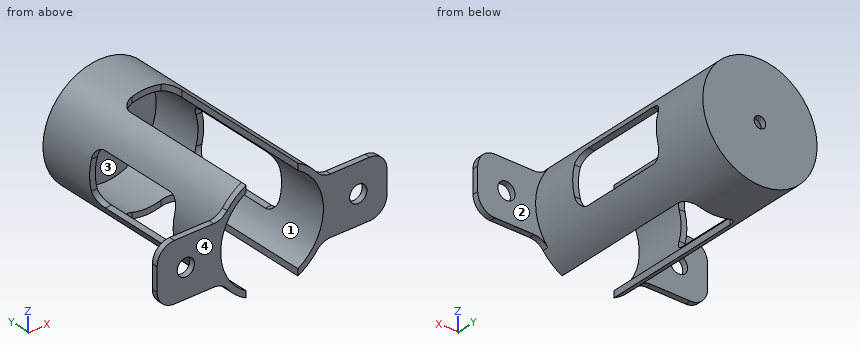
from build123d import *

# Parameters (mm, degrees)
SKETCH2_R           = 9.9375
BOSS_EXTRUDE1_DEPTH = 35.384
SKETCH4_R           = 1
CUT_EXTRUDE2_DEPTH  = 39.072762817
BOSS_EXTRUDE2_START = 1
SKETCH11_R          = 8.9375
BOSS_EXTRUDE2_DEPTH = 1
SKETCH12_R          = 8.9375
CUT_EXTRUDE7_DEPTH  = 34.384
CUT_EXTRUDE8_START  = -1
CUT_EXTRUDE8_DEPTH  = 26.538
SKETCH14_W          = 9
SKETCH14_H          = 17.692
CUT_EXTRUDE9_DEPTH  = 63.054664307
FILLET3_R           = 2
FILLET4_R           = 3
CUT_EXTRUDE10_REACH = 43.842
SKETCH15_R          = 1.5


# Read off the part's stored shape, not the designer's step: Cut-Extrude8
with BuildPart() as part:
    # Sketch2 → Boss-Extrude1 (new body)
    with BuildSketch(Plane(origin=(0, 0, 0), x_dir=(1, 0, 0), z_dir=(0, 1, 0))):
        with Locations(Location((0, 0, 0), (0, 0, 270))):
            Circle(SKETCH2_R)
    extrude(amount=BOSS_EXTRUDE1_DEPTH)

    # Sketch4 → Cut-Extrude2 (cut, through all)
    with BuildSketch(Plane(origin=(0, 35.384, 0), x_dir=(1, 0, 0), z_dir=(0, 1, 0))):
        with Locations(Location((0, 0, 0), (0, 0, 270))):
            Circle(SKETCH4_R)
    extrude(amount=-CUT_EXTRUDE2_DEPTH, mode=Mode.SUBTRACT)

    # Sketch11 → Boss-Extrude2 (add)
    with BuildSketch(Plane.XZ.offset(BOSS_EXTRUDE2_START)):
        with BuildLine():
            Line((8.588009446, 5), (20, 5))
            Line((20, 5), (20, -5))
            Line((20, -5), (8.588009446, -5))
            ThreePointArc((8.588009446, -5), (0, -9.9375), (-8.588009446, -5))
            Line((-8.588009446, -5), (-20, -5))
            Line((-20, -5), (-20, 5))
            Line((-20, 5), (-8.588009446, 5))
            ThreePointArc((-8.588009446, 5), (0, 9.9375), (8.588009446, 5))
        make_face()
        with Locations(Location((0, 0, 0), (0, 0, 270))):
            Circle(SKETCH11_R, mode=Mode.SUBTRACT)
    extrude(amount=-BOSS_EXTRUDE2_DEPTH)

    # Sketch12 → Cut-Extrude7 (cut)
    with BuildSketch(Plane.XZ):
        with Locations(Location((0, 0, 0), (0, 0, 270))):
            Circle(SKETCH12_R)
    extrude(amount=-CUT_EXTRUDE7_DEPTH, mode=Mode.SUBTRACT)

    # Cut-Extrude8 outline → Cut-Extrude8 (cut)
    with BuildSketch(Plane(origin=(0, 0, 0), x_dir=(1, 0, 0), z_dir=(0, 1, 0)).offset(CUT_EXTRUDE8_START)):
        with BuildLine():
            ThreePointArc((4.5, -7.721975541), (0, -8.9375), (-4.5, -7.721975541))
            Line((-4.5, -7.721975541), (-4.5, -8.860243013))
            ThreePointArc((-4.5, -8.860243013), (0, -9.9375), (4.5, -8.860243013))
            Line((4.5, -8.860243013), (4.5, -7.721975541))
        make_face()
        with BuildLine():
            Line((-4.5, 8.860243013), (-4.5, 7.721975541))
            ThreePointArc((-4.5, 7.721975541), (0, 8.9375), (4.5, 7.721975541))
            Line((4.5, 7.721975541), (4.5, 8.860243013))
            ThreePointArc((4.5, 8.860243013), (0, 9.9375), (-4.5, 8.860243013))
        make_face()
    extrude(amount=CUT_EXTRUDE8_DEPTH, mode=Mode.SUBTRACT)

    # Sketch14 → Cut-Extrude9 (cut, through all)
    with BuildSketch(Plane(origin=(30, 0, 0), x_dir=(0, 0, -1), z_dir=(1, 0, 0))):
        with Locations((0, 16.692)):
            Rectangle(SKETCH14_W, SKETCH14_H)
    extrude(amount=-CUT_EXTRUDE9_DEPTH, mode=Mode.SUBTRACT)

    # Fillet3
    fillet3_edges = [part.edges().sort_by_distance(p)[0] for p in [
        (4.5, 25.538, 8.291109277),
        (4.5, 25.538, -8.291109277),
        (-4.5, 25.538, -8.291109277),
        (-4.5, 25.538, 8.291109277),
        (8.291109277, 25.538, -4.5),
        (-8.291109277, 25.538, -4.5),
        (8.291109277, 7.846, -4.5),
        (-8.291109277, 7.846, -4.5),
        (-8.291109277, 7.846, 4.5),
        (8.291109277, 7.846, 4.5),
        (8.291109277, 25.538, 4.5),
        (-8.291109277, 25.538, 4.5),
    ]]
    fillet(fillet3_edges, radius=FILLET3_R)

    # Fillet4
    # the kernel refuses this fillet: 3 mm, written as the material it adds along each edge
    with BuildSketch(Plane(origin=(8.588009446, -1, -5), x_dir=(-0.562116261978449, 0, -0.8270582252897166), z_dir=(0, 1, 0)), Plane(origin=(-8.588009446, -1, 5), x_dir=(0.5621162619784511, 0, 0.8270582252897152), z_dir=(0, 1, 0))) as fillet4_piece_1:
        with BuildLine():
            CenterArc((1.593293854, -2.992714011), FILLET4_R, 93.994010432, 51.803711499)
            Line((-0.887880822, -1.306365225), (0, 0))
            ThreePointArc((0, 0), (0.692168641, -0.024134839), (1.384337283, 0))
        make_face()
    extrude(amount=1)
    with BuildSketch(Plane(origin=(8.588009446, -1, 5), x_dir=(-0.5621162619784463, 0, 0.8270582252897184), z_dir=(0, 1, 0)), Plane(origin=(-8.588009446, -1, -5), x_dir=(0.5621162619784531, 0, -0.8270582252897138), z_dir=(0, 1, 0))) as fillet4_piece_2:
        with BuildLine():
            CenterArc((1.593293854, 2.992714011), FILLET4_R, 214.20227807, 51.803711499)
            Line((-0.887880822, 1.306365225), (0, 0))
            ThreePointArc((0, 0), (0.692168641, 0.024134839), (1.384337283, 0))
        make_face()
    extrude(amount=1)
    # the kernel refuses this fillet: 3 mm, written as the material it takes off along each edge
    with BuildSketch(Plane(origin=(20, -8.5, -5), x_dir=(0, 0, 1), z_dir=(0, 1, 0)), Plane(origin=(20, -8.5, 5), x_dir=(-1, 0, 0), z_dir=(0, 1, 0))) as fillet4_2_piece_1:
        with BuildLine():
            CenterArc((FILLET4_R, -FILLET4_R), FILLET4_R, 90, 90)
            Line((0, -FILLET4_R), (0, 0))
            Line((0, 0), (FILLET4_R, 0))
        make_face()
    extrude(amount=16, mode=Mode.SUBTRACT)
    with BuildSketch(Plane(origin=(-20, -8.5, 5), x_dir=(1, 0, 0), z_dir=(0, 1, 0)), Plane(origin=(-20, -8.5, -5), x_dir=(0, 0, 1), z_dir=(0, 1, 0))) as fillet4_2_piece_2:
        with BuildLine():
            CenterArc((FILLET4_R, FILLET4_R), FILLET4_R, 180, 90)
            Line((0, FILLET4_R), (0, 0))
            Line((0, 0), (FILLET4_R, 0))
        make_face()
    extrude(amount=16, mode=Mode.SUBTRACT)

    # Sketch15 → Cut-Extrude10 (cut, up to next)
    with BuildSketch(Plane(origin=(0, 0, 0), x_dir=(1, 0, 0), z_dir=(0, 1, 0)), mode=Mode.PRIVATE) as cut_extrude10_sk1:
        with Locations(Location((-15, 0, 0), (0, 0, 270))):
            Circle(SKETCH15_R)
    cut_extrude10_tool1 = extrude(cut_extrude10_sk1.sketch, amount=-CUT_EXTRUDE10_REACH, mode=Mode.PRIVATE) & part.part
    # Sketch15 → Cut-Extrude10 (cut, up to next)
    with BuildSketch(Plane(origin=(0, 0, 0), x_dir=(1, 0, 0), z_dir=(0, 1, 0)), mode=Mode.PRIVATE) as cut_extrude10_sk2:
        with Locations(Location((15, 0, 0), (0, 0, 270))):
            Circle(SKETCH15_R)
    cut_extrude10_tool2 = extrude(cut_extrude10_sk2.sketch, amount=-CUT_EXTRUDE10_REACH, mode=Mode.PRIVATE) & part.part
    add(cut_extrude10_tool1.solids().sort_by_distance((-15, 0, 0))[0], mode=Mode.SUBTRACT)
    add(cut_extrude10_tool2.solids().sort_by_distance((15, 0, 0))[0], mode=Mode.SUBTRACT)


solid = part.part
The listing builds one solid part. Answer for the finished solid, in the listing's coordinates (mm). Face numbers are marked on the shaded views. A direction names the side the tool comes from. Round coordinates to 2 decimals unless told otherwise and drop trailing zeros. Write each loop counter-clockwise with the first axis right and the second up, starting at its lowest first coordinate (ties: lowest second). Pieces come first, ordered by that corner, then holes. Notation, with made-up numbers: M 13.5,5 L 56.5,5 A17 ccw 56.5,13 Z; hole C 71.25,81.25 d2. An arc over 180 degrees is marked long. Write each question's results on one line, items separated by ' | '. Start each with the question number.
(1) The part is cut by section B-B, the plane y = 20. Write down the section's boundary in (x, z) (1 decimal), and give its area (3 significant figures).
(2) The part is cut by section A-A, the plane z = 0. Give the number of separate pieces and of enclosed holes in the cut face, and give its area (3 significant figures).
(3) Find the intervals of material crossed by line 1 (X direction, y = -0.45, z = 0); line 2 (X direction, y = 34.85, z = 0); line 3 (Y direction, x = -0.5, z = -7.5), in increasing order.
(4) For the marked faces 3 and 4, determine the directions among +Z, -Z, +X, -X, +Y, -Y from which every point of the face is accessible in a straight line to the end or side of a thin tool.
(5) The part is cut by section C-C, the plane y = 6. Write down the section's boundary in (x, z) (1 decimal), and give its area (3 significant figures).
(6) The part is cut by section D-D, the plane x = 0. Write down the section's boundary in (y, z).
(7) Each of these flat-tipped pins is pushed along its axis until it touches: P1, Ø1, axis at x = 8.5, y = 12.5, coming from the -Z side; P2, Ø3, axis at y = 3, z = -1, coming from the +X side; P3, Ø1.6, axis at x = 0, z = 0, coming from the +Y side; P4, Ø0.6, axis at y = 6, z = 8, coming from the +X side. Where does it stop, or does it pass through?
(8) Determine the mould class of the marked faces 1 and 2 for opening direction X: +X half, -X half, draft (parallel to the pull), parting line (faces both ways), or undercut.
Worked answers:
1) outline: M -8.9,-4.5 A9.9 ccw -4.5,-8.9 L -4.5,-7.7 A8.9 cw -7.7,-4.5 Z; M -8.9,4.5 L -7.7,4.5 A8.9 cw -4.5,7.7 L -4.5,8.9 A9.9 ccw Z; M 4.5,-8.9 A9.9 ccw 8.9,-4.5 L 7.7,-4.5 A8.9 cw 4.5,-7.7 Z; M 4.5,7.7 A8.9 cw 7.7,4.5 L 8.9,4.5 A9.9 ccw 4.5,8.9 Z | area: 21.8 mm²
2) separate pieces: 6 | enclosed holes: 0 | area: 67.4 mm²
3) line 1: x = -20 to -16.5, -13.5 to -8.94, 8.94 to 13.5, 16.5 to 20 | line 2: x = -9.94 to -1, 1 to 9.94 | line 3: y = 34.38 to 35.38
4) face 3: -Y | face 4: +Z, -Z, +X, -X, -Y
5) outline: M -4.5,-8.9 L -4.5,-7.7 A8.9 cw -4.5,7.7 L -4.5,8.9 A9.9 ccw Z; M 4.5,-8.9 A9.9 ccw 4.5,8.9 L 4.5,7.7 A8.9 cw 4.5,-7.7 Z | area: 40.5 mm²
6) outline: M 25.54,-9.94 L 35.38,-9.94 L 35.38,-1 L 34.38,-1 L 34.38,-8.94 L 25.54,-8.94 Z; M 25.54,8.94 L 34.38,8.94 L 34.38,1 L 35.38,1 L 35.38,9.94 L 25.54,9.94 Z
7) P1: stops at z = -5.9 | P2: stops at x = 9.94 | P3: passes through | P4: stops at x = 6.28
8) face 1: undercut | face 2: draft
